Here's how the part is built. I have some questions about the finished solid (model axes, mm). Face numbers are marked on the shaded views. A direction names the side the tool comes from. Coordinates: 2 decimals unless noted, no trailing zeros. Use one line per item in the form item = value. Start each with the question number.
(1) Will these pins go through, and if not, where does the flat tip stop? P1, Ø5.5, axis at y = 36.5, z = 71, coming from the +X side; P2, Ø9, axis at x = -36.5, y = 34.5, coming from the +Z side; P3, Ø3, axis at x = -37, y = 5, coming from the -Z side.
(2) Please list where these lines run through material, in increasing order: L1, parallel to Y at x = -68, z = 8.5; L2, parallel to Z at x = -71.5, y = 40.5; L3, parallel to Y at x = -63.5, z = 21.5.
(3) On a 3-axis mill with a long thin cutter (end or side, diameter ignored), from which of +Z, -Z, +X, -X, +Y, -Y can I reach the whole of each face in a straight line? I mean the marked faces 1, 2 and 3. Say none if no direction works.
(4) Imagine slicing it at A-A, the plane y = 24.5. State how many separate pieces and enclosed holes the cut face has, and give its area (3 significant figures).
(5) Thinking about a two-plate mould opening in Y: for the marked faces 4, 5 and 6, which applies, +Y half, -Y half, draft (parallel to the pull), parting line (faces both ways), or undercut?
```python
from build123d import *

# Parameters (mm, degrees)
F1_DEPTH  = 25.4
F2_R      = 25.39999
F3_R      = 30.0176409496
F4_DEPTH  = 3.81
F5_R      = 35.0976409496
F6_DEPTH  = 6.35
F7_R      = 35.0976409496
F8_DEPTH  = 10.16
F9_DEPTH  = 10.16
F10_W     = 38.3836512671
F10_H     = 10.16
F11_DEPTH = 15.24
F12_R     = 3.0425051658
F13_DEPTH = 31.75
F12_R_2   = 1.8599906357
F12_R_3   = 2.469076523
F12_R_4   = 2.4371339636
F12_W     = 11.43
F12_H     = 11.43
F15_DEPTH = 7.62
F18_DEPTH = 6.35


# Not quite as in the source:
# - a fillet or chamfer is up to 0.001 mm smaller than in the source, because OpenCascade refuses the exact size


with BuildPart() as f1:
    # F0 (on Front) → F1 (new body)
    with BuildSketch(Plane.XZ):
        with BuildLine():
            ThreePointArc((-51.3157695532, 20.9789809584), (-28.7430536644, 30.3289060191), (-19.3931286036, 52.9016219079))
            ThreePointArc((-19.3931286036, 52.9016219079), (-73.888485442, 75.4743377968), (-51.3157695532, 20.9789809584))
        make_face()
    extrude(amount=F1_DEPTH)

    # F2 (radius 25.4 in the source; OpenCascade refuses exactly that, so slightly less here)
    f2_edges = [f1.edges().sort_by_distance(p)[0] for p in [
        (-51.31577, -25.4, 84.824263),
    ]]
    fillet(f2_edges, radius=F2_R)

    # F3 (on face) → F4 (join)
    with BuildSketch(Plane(origin=(0, 0, 0), x_dir=(-1, 0, 0), z_dir=(0, 1, 0))):
        with Locations((51.3157695532, 52.9016219079)):
            Circle(F3_R)
    extrude(amount=F4_DEPTH)

    # F5 (on face) → F6 (join)
    with BuildSketch(Plane(origin=(0, 3.81, 0), x_dir=(-1, 0, 0), z_dir=(0, 1, 0))):
        with Locations((51.3157695532, 52.9016219079)):
            Circle(F5_R)
    extrude(amount=F6_DEPTH)



with BuildPart() as f8:
    # F7 (on face) → F8 (new body)
    with BuildSketch(Plane(origin=(0, 10.16, 0), x_dir=(-1, 0, 0), z_dir=(0, 1, 0))):
        with BuildLine():
            Line((32.1239439196, 16.1649812187), (70.5075951867, 16.1649812187))
            ThreePointArc((70.5075951867, 16.1649812187), (51.3157695532, 94.3492628575), (32.1239439196, 16.1649812187))
        make_face()
        with Locations((51.3157695532, 52.9016219079)):
            Circle(F7_R, mode=Mode.SUBTRACT)
    extrude(amount=F8_DEPTH)


with BuildPart() as f1_1:
    add(f1.part)

    add(f8.part)  # F9 merges F8
    # F7 (on face) → F9 (join)
    with BuildSketch(Plane(origin=(0, 10.16, 0), x_dir=(-1, 0, 0), z_dir=(0, 1, 0))):
        with Locations((51.3157695532, 52.9016219079)):
            Circle(F7_R)
    extrude(amount=F9_DEPTH)

    # F10 (on face) → F11 (join)
    with BuildSketch(Plane(origin=(0, 0, 16.1649812187), x_dir=(1, 0, 0), z_dir=(0, 0, -1))):
        with Locations((-51.3157695532, -15.24)):
            Rectangle(F10_W, F10_H)
    extrude(amount=F11_DEPTH)

    # F12 (on face) → F13, piece 2 (join)
    with BuildSketch(Plane(origin=(0, 20.32, 0), x_dir=(-1, 0, 0), z_dir=(0, 1, 0))):
        with Locations((67.4533173442, 4.8855347559)):
            Circle(F12_R_2)
        with Locations((35.3975147009, 4.8855352215)):
            Circle(F12_R_2)
        with Locations((39.9559102952, 4.8855347559)):
            Circle(F12_R_2)
        with Locations((44.3672593683, 4.8855361529)):
            Circle(F12_R_2)
        with Locations((49.0726977587, 4.8855366185)):
            Circle(F12_R_2)
        with Locations((53.6310952157, 4.8855361529)):
            Circle(F12_R_2)
        with Locations((58.0424424261, 4.8855347559)):
            Circle(F12_R_2)
        with Locations((62.6008361578, 4.8855366185)):
            Circle(F12_R_2)
        with Locations((35.3975147009, 11.7231269833)):
            Circle(F12_R_3)
        with Locations((67.4533173442, 11.7966495454)):
            Circle(F12_R_4)
        with Locations((13.5955894366, 59.4231709838)):
            Circle(F12_R)
        with Locations((50.6292656064, 91.1249816418)):
            Circle(F12_R)
        with Locations((18.5757915024, 33.1017822027)):
            Circle(F12_R)
        with Locations((25.7929724175, 81.4013928175)):
            Circle(F12_R)
        with Locations((89.0821111389, 59.1946728528)):
            Circle(F12_R)
        with Locations((84.0856006835, 33.2405753434)):
            Circle(F12_R)
        with Locations((76.2026160955, 81.9760784507)):
            Circle(F12_R)
        with Locations((36.2023725174, 88.0633927882)):
            Circle(F12_R)
        with Locations((88.8045257889, 45.3154779971)):
            Circle(F12_R)
        with Locations((18.0206210352, 71.6859512031)):
            Circle(F12_R)
        with Locations((13.761004433, 45.646622777)):
            Circle(F12_R)
        with Locations((64.6823644638, 88.7463241816)):
            Circle(F12_R)
        with Locations((84.7154408693, 71.5908780694)):
            Circle(F12_R)
        with Locations((26.7645169515, 23.525133729)):
            Circle(F12_R)
        with Locations((76.0732889175, 23.7615462393)):
            Circle(F12_R)
        with Locations((68.7132014135, 68.4635355137)):
            Rectangle(F12_W, F12_H)
        with Locations((33.9833064711, 37.3775935507)):
            Rectangle(F12_W, F12_H)
        with Locations((33.9119490236, 68.4635355137)):
            Rectangle(F12_W, F12_H)
        with Locations((68.7132014135, 37.3397083022)):
            Rectangle(F12_W, F12_H)
        with Locations((33.9833064711, 48.6564002931)):
            Circle(F12_R)
        with Locations((33.9119490236, 57.7810369432)):
            Circle(F12_R)
        with Locations((56.8348169327, 68.4635355137)):
            Circle(F12_R)
        with Locations((68.7132014135, 57.3359318078)):
            Circle(F12_R)
        with Locations((68.7132014135, 48.6564002931)):
            Circle(F12_R)
        with Locations((55.7220578194, 37.3397083022)):
            Circle(F12_R)
        with Locations((47.0425225794, 68.4635355137)):
            Circle(F12_R)
        with Locations((45.2621094882, 37.3775935507)):
            Circle(F12_R)
    extrude(amount=F13_DEPTH)

    # F14 (on face) → F15 (join)
    with BuildSketch(Plane(origin=(0, 52.07, 0), x_dir=(-1, 0, 0), z_dir=(0, 1, 0))):
        with BuildLine():
            Line((70.5171748996, 16.2905004551), (70.5051029675, 16.2905004551))
            ThreePointArc((70.5051029675, 16.2905004551), (51.313277334, 94.474782094), (32.1214517004, 16.2905004551))
            Line((32.1214517004, 16.2905004551), (32.1214517004, 1.0184145067))
            Line((32.1214517004, 1.0184145067), (70.5171748996, 1.0184145067))
            Line((70.5171748996, 1.0184145067), (70.5171748996, 16.2905004551))
        make_face()
    extrude(amount=F15_DEPTH)

    # F17 (on face) → F18 (join)
    with BuildSketch(Plane(origin=(0, 59.69, 0), x_dir=(-1, 0, 0), z_dir=(0, 1, 0))):
        with BuildLine():
            Line((77.230297029, -5.3806910291), (77.230297029, 10.8189785437))
            ThreePointArc((77.230297029, 10.8189785437), (51.3255716567, 102.5571396186), (25.3753070366, 10.8318499752))
            Line((25.3753070366, 10.8318499752), (25.3753070366, -5.3806910291))
            Line((25.3753070366, -5.3806910291), (77.230297029, -5.3806910291))
        make_face()
    extrude(amount=F18_DEPTH)


with BuildPart() as f13:
    # F12 (on face) → F13 (new body)
    with BuildSketch(Plane(origin=(0, 20.32, 0), x_dir=(-1, 0, 0), z_dir=(0, 1, 0))):
        with Locations((853.825874161, 233.101002872)):
            Circle(F12_R)
    extrude(amount=F13_DEPTH)


solid = f1_1.part
```
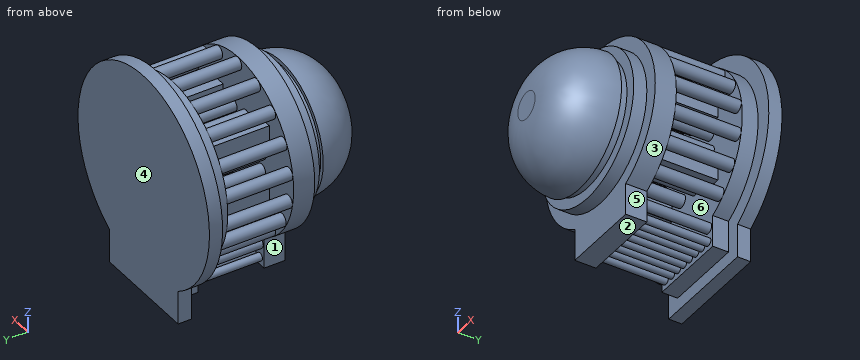
Answer:
q1.P1 = -14.98
q1.P2 = 91.11
q1.P3 = 20.23
q2.L1 = 10.16 to 20.32, 52.07 to 66.04
q2.L2 = 31.62 to 43.05, 47.44 to 49.88, 56.12 to 58.56, 62.75 to 74.18
q2.L3 = 3.81 to 20.32, 52.07 to 66.04
q3.face_1 = -Z, -X, -Y
q3.face_2 = -Z, +X, -X, -Y
q3.face_3 = -Y
q4.separate_pieces = 37
q4.enclosed_holes = 0
q4.area = 1,320 mm²
q5.face_4 = +Y half
q5.face_5 = draft
q5.face_6 = undercut
